The model under review builds one solid part; all positions refer to its coordinate system, in mm. Face numbers are marked on the shaded views. A direction names the side the tool comes from. Round coordinates to 2 decimals unless told otherwise and drop trailing zeros. Loops run counter-clockwise (first coordinate to the right, second up) from the corner with the lowest first, then second, coordinate; pieces in that order, holes last. Notation, with made-up numbers: (50.25, -32) - (58.25, -32) arc R23 cw to (58.25, -11) - close; hole circle Ø7 at (-4.75, -34). An arc over 180 degrees is marked (long way). Answer as CSV lines item,"result".
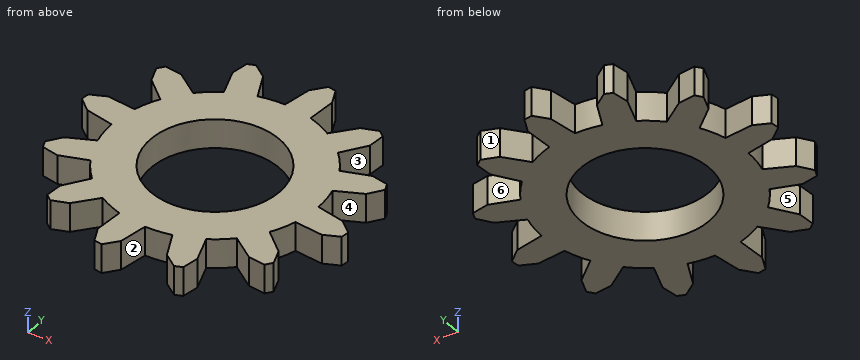
from build123d import *

# Parameters (mm, degrees)
F0_R     = 11
F1_DEPTH = 5


with BuildPart() as f1:
    # F0 (on Top) → F1 (new body)
    with BuildSketch(Plane.XY):
        with BuildLine():
            ThreePointArc((16.8326, -4.786812), (17.332347, -2.416557), (17.5, 0))
            ThreePointArc((17.5, 0), (17.367213, 2.151727), (16.970865, 4.2708))
            ThreePointArc((16.970865, 4.2708), (16.218531, 6.573374), (15.155445, 8.75))
            ThreePointArc((15.155445, 8.75), (13.964584, 10.547056), (12.561801, 12.184054))
            ThreePointArc((12.561801, 12.184054), (10.758973, 13.801974), (8.75, 15.155445))
            ThreePointArc((8.75, 15.155445), (6.820156, 16.116311), (4.786812, 16.8326))
            ThreePointArc((4.786812, 16.8326), (2.416557, 17.332347), (0, 17.5))
            ThreePointArc((0, 17.5), (-2.151727, 17.367213), (-4.2708, 16.970865))
            ThreePointArc((-4.2708, 16.970865), (-6.573374, 16.218531), (-8.75, 15.155445))
            ThreePointArc((-8.75, 15.155445), (-10.547056, 13.964584), (-12.184054, 12.561801))
            ThreePointArc((-12.184054, 12.561801), (-13.801974, 10.758973), (-15.155445, 8.75))
            ThreePointArc((-15.155445, 8.75), (-16.116311, 6.820156), (-16.8326, 4.786812))
            ThreePointArc((-16.8326, 4.786812), (-17.332347, 2.416557), (-17.5, 0))
            ThreePointArc((-17.5, 0), (-17.367213, -2.151727), (-16.970865, -4.2708))
            ThreePointArc((-16.970865, -4.2708), (-16.218531, -6.573374), (-15.155445, -8.75))
            ThreePointArc((-15.155445, -8.75), (-13.964584, -10.547056), (-12.561801, -12.184054))
            ThreePointArc((-12.561801, -12.184054), (-10.758973, -13.801974), (-8.75, -15.155445))
            ThreePointArc((-8.75, -15.155445), (-6.820156, -16.116311), (-4.786812, -16.8326))
            ThreePointArc((-4.786812, -16.8326), (-2.416557, -17.332347), (0, -17.5))
            ThreePointArc((0, -17.5), (2.151727, -17.367213), (4.2708, -16.970865))
            ThreePointArc((4.2708, -16.970865), (6.573374, -16.218531), (8.75, -15.155445))
            ThreePointArc((8.75, -15.155445), (10.547056, -13.964584), (12.184054, -12.561801))
            ThreePointArc((12.184054, -12.561801), (13.801974, -10.758973), (15.155445, -8.75))
            ThreePointArc((15.155445, -8.75), (16.116311, -6.820156), (16.8326, -4.786812))
        make_face()
        Circle(F0_R, mode=Mode.SUBTRACT)
        with BuildLine():
            Line((22.193341, -0.890096), (17.5, 0))
            ThreePointArc((17.5, 0), (17.332347, -2.416557), (16.8326, -4.786812))
            Line((16.8326, -4.786812), (21.59042, -5.214441))
            Line((21.59042, -5.214441), (24.161443, -4.058901))
            ThreePointArc((24.161443, -4.058901), (24.265286, -3.38318), (24.350235, -2.704824))
            Line((24.350235, -2.704824), (22.193341, -0.890096))
        make_face()
        with BuildLine():
            ThreePointArc((15.155445, 8.75), (16.218531, 6.573374), (16.970865, 4.2708))
            Line((16.970865, 4.2708), (21.305073, 6.279372))
            Line((21.305073, 6.279372), (22.953874, 8.56561))
            ThreePointArc((22.953874, 8.56561), (22.705944, 9.202724), (22.440334, 9.832671))
            Line((22.440334, 9.832671), (19.665045, 10.325825))
            Line((19.665045, 10.325825), (15.155445, 8.75))
        make_face()
        with BuildLine():
            Line((18.774949, -11.867516), (15.155445, -8.75))
            ThreePointArc((15.155445, -8.75), (13.801974, -10.758973), (12.184054, -12.561801))
            Line((12.184054, -12.561801), (16.090632, -15.311048))
            Line((16.090632, -15.311048), (18.894973, -15.595833))
            ThreePointArc((18.894973, -15.595833), (19.322764, -15.062562), (19.73551, -14.517564))
            Line((19.73551, -14.517564), (18.774949, -11.867516))
        make_face()
        with BuildLine():
            ThreePointArc((8.75, 15.155445), (10.758973, 13.801974), (12.561801, 12.184054))
            Line((12.561801, 12.184054), (15.311048, 16.090632))
            Line((15.311048, 16.090632), (15.595833, 18.894973))
            ThreePointArc((15.595833, 18.894973), (15.062562, 19.322764), (14.517564, 19.73551))
            Line((14.517564, 19.73551), (11.867516, 18.774949))
            Line((11.867516, 18.774949), (8.75, 15.155445))
        make_face()
        with BuildLine():
            Line((10.325825, -19.665045), (8.75, -15.155445))
            ThreePointArc((8.75, -15.155445), (6.573374, -16.218531), (4.2708, -16.970865))
            Line((4.2708, -16.970865), (6.279372, -21.305073))
            Line((6.279372, -21.305073), (8.56561, -22.953874))
            ThreePointArc((8.56561, -22.953874), (9.202724, -22.705944), (9.832671, -22.440334))
            Line((9.832671, -22.440334), (10.325825, -19.665045))
        make_face()
        with BuildLine():
            ThreePointArc((0, 17.5), (2.416557, 17.332347), (4.786812, 16.8326))
            Line((4.786812, 16.8326), (5.214441, 21.59042))
            Line((5.214441, 21.59042), (4.058901, 24.161443))
            ThreePointArc((4.058901, 24.161443), (3.38318, 24.265286), (2.704824, 24.350235))
            Line((2.704824, 24.350235), (0.890096, 22.193341))
            Line((0.890096, 22.193341), (0, 17.5))
        make_face()
        with BuildLine():
            Line((-0.890096, -22.193341), (0, -17.5))
            ThreePointArc((0, -17.5), (-2.416557, -17.332347), (-4.786812, -16.8326))
            Line((-4.786812, -16.8326), (-5.214441, -21.59042))
            Line((-5.214441, -21.59042), (-4.058901, -24.161443))
            ThreePointArc((-4.058901, -24.161443), (-3.38318, -24.265286), (-2.704824, -24.350235))
            Line((-2.704824, -24.350235), (-0.890096, -22.193341))
        make_face()
        with BuildLine():
            ThreePointArc((-8.75, 15.155445), (-6.573374, 16.218531), (-4.2708, 16.970865))
            Line((-4.2708, 16.970865), (-6.279372, 21.305073))
            Line((-6.279372, 21.305073), (-8.56561, 22.953874))
            ThreePointArc((-8.56561, 22.953874), (-9.202724, 22.705944), (-9.832671, 22.440334))
            Line((-9.832671, 22.440334), (-10.325825, 19.665045))
            Line((-10.325825, 19.665045), (-8.75, 15.155445))
        make_face()
        with BuildLine():
            Line((-11.867516, -18.774949), (-8.75, -15.155445))
            ThreePointArc((-8.75, -15.155445), (-10.758973, -13.801974), (-12.561801, -12.184054))
            Line((-12.561801, -12.184054), (-15.311048, -16.090632))
            Line((-15.311048, -16.090632), (-15.595833, -18.894973))
            ThreePointArc((-15.595833, -18.894973), (-15.062562, -19.322764), (-14.517564, -19.73551))
            Line((-14.517564, -19.73551), (-11.867516, -18.774949))
        make_face()
        with BuildLine():
            ThreePointArc((-15.155445, 8.75), (-13.801974, 10.758973), (-12.184054, 12.561801))
            Line((-12.184054, 12.561801), (-16.090632, 15.311048))
            Line((-16.090632, 15.311048), (-18.894973, 15.595833))
            ThreePointArc((-18.894973, 15.595833), (-19.322764, 15.062562), (-19.73551, 14.517564))
            Line((-19.73551, 14.517564), (-18.774949, 11.867516))
            Line((-18.774949, 11.867516), (-15.155445, 8.75))
        make_face()
        with BuildLine():
            Line((-19.665045, -10.325825), (-15.155445, -8.75))
            ThreePointArc((-15.155445, -8.75), (-16.218531, -6.573374), (-16.970865, -4.2708))
            Line((-16.970865, -4.2708), (-21.305073, -6.279372))
            Line((-21.305073, -6.279372), (-22.953874, -8.56561))
            ThreePointArc((-22.953874, -8.56561), (-22.705944, -9.202724), (-22.440334, -9.832671))
            Line((-22.440334, -9.832671), (-19.665045, -10.325825))
        make_face()
        with BuildLine():
            ThreePointArc((-17.5, 0), (-17.332347, 2.416557), (-16.8326, 4.786812))
            Line((-16.8326, 4.786812), (-21.59042, 5.214441))
            Line((-21.59042, 5.214441), (-24.161443, 4.058901))
            ThreePointArc((-24.161443, 4.058901), (-24.265286, 3.38318), (-24.350235, 2.704824))
            Line((-24.350235, 2.704824), (-22.193341, 0.890096))
            Line((-22.193341, 0.890096), (-17.5, 0))
        make_face()
    extrude(amount=F1_DEPTH)


solid = f1.part
1. Clearance check with flat-ended pins moving along their axes: pin 1 (3 mm diameter, centred on y = 16.5, z = 4, fed in from +X); pin 2 (3 mm diameter, centred on y = 9.5, z = 4.5, fed in from -X); pin 3 (1 mm diameter, centred on x = 5, z = 1.5, fed in from -Y). State where each tip first meets the part, or that it passes through.
Numbers:
pin 1,"stops at x = 15.5"
pin 2,"stops at x = -17.77"
pin 3,"stops at y = -19.62"
2. Wall thickness on probe 1 along X at (y, z) = (7, 2.7); probe 2 along X at (y, z) = (22, 2.8); probe 3 along Y at (x, z) = (2, 1.8): over which ranges is each line inside the solid? List them lowest first.
Numbers:
probe 1,"x = -16.04 to -8.49, 8.49 to 21.82"
probe 2,"x = -9.91 to -7.24, 0.85 to 5.03"
probe 3,"y = -17.39 to -10.82, 10.82 to 23.51"
3. Draft analysis for pull direction X (two halves, no side actions). For the marked faces 4, 5 and 6, state which applies: +X half, -X half, draft (parallel to the pull), parting line (faces both ways), or undercut.
Numbers:
face 4,"+X half"
face 5,"-X half"
face 6,"undercut"
4. Tool access review of the marked faces 1, 2 and 3: name each direction out of +Z, -Z, +X, -X, +Y, -Y from which nothing blocks a thin tool from reaching the whole face with its end or side.
Numbers:
face 1,"+Z, -Z, +Y"
face 2,"+Z, -Z, -Y"
face 3,"+Z, -Z, +X"
5. Take a section at B-B (x = -3.5). State the section outline as (y, z) points.
Numbers:
outline,"(-24.25, 0) - (-10.43, 0) - (-10.43, 5) - (-24.25, 5) - close; (10.43, 0) - (17.15, 0) - (17.15, 5) - (10.43, 5) - close"
6. Take a section at A-A (y = -7). State the section outline as (x, z) points, plus the area to 3 significant figures.
Numbers:
outline,"(-21.82, 0) - (-8.49, 0) - (-8.49, 5) - (-21.82, 5) - close; (8.49, 0) - (16.04, 0) - (16.04, 5) - (8.49, 5) - close"
area,"104 mm²"
